Here's how the part is built. I have some questions about the finished solid (model axes, mm). A direction names the side the tool comes from. Coordinates: 2 decimals unless noted, no trailing zeros. Order: outer loops, then holes, each group sorted by start corner. A loop starts at its lowest first (then second) coordinate and runs counter-clockwise, first axis right, second up. Notation, with made-up numbers: (35, 20.25) - (78, 20.25) arc R17 cw to (78, 51.25) - close; hole circle Ø11 at (-38.75, 9). An arc over 180 degrees is marked (long way). Answer in a Markdown table with one row per item. Add a question column.
Item 1: Thinking about a two-plate mould opening in X: for faces 3 (the flat face through (-72.283, -3.131, 117.315)), 4 (the cylindrical face through (-72.839, -3.219, 88.523)), 5 (the flat face through (71.426, -3.131, 119.51)), 6 (the flat face through (-1, -3, 200)), which applies, +X half, -X half, draft (parallel to the pull), parting line (faces both ways), or undercut?
Item 2: I want a section at D-D (y = -3.25). Count the separate pieces of the cut face and the enclosed holes in it, plus the area to 3 significant figures.
Item 3: If I drill on line 1 along X through (y, z) = (-1.75, 90); line 2 along X through (y, z) = (-1.5, 16.5); line 3 along X through (y, z) = (-0.75, -13), over which ranges is the centre line in solid material (lowest first)? Write a range as from..to.
Item 4: On a 3-axis mill with a long thin cutter (end or side, diameter ignored), from which of +Z, -Z, +X, -X, +Y, -Y can I reach the whole of each face in a straight line? I mean faces 1 (the flat face through (-2, 0, 77)), 2 (the flat face through (0, -3, 170)). Say none if no direction works.
Item 5: I want a section at B-B (z = 133). Please give me the cut outline in (x, y), plus the area to 3 significant figures.
Item 6: Will these pins go through, and if not, where does the flat tip stop? pin 1 Ø4 at (x, z) = (-30, 190) entering from +Y; pin 2 Ø6.5 at (x, z) = (70.64, 70.64) entering from -Y; pin 3 Ø3 at (x, y) = (-62, -2) entering from -Z; pin 4 Ø1 at (y, z) = (-4, 37.5) entering from +X.
Item 7: I want a section at C-C (z = -15.5). Please give me the cut outline in (x, y), plus the area to 3 significant figures.
Item 8: I want a section at A-A (x = 0). Please give me the cut outline in (y, z), plus the area to 3 significant figures.
```python
from build123d import *

# Parameters (mm, degrees)
BOSS_EXTRUDE1_DEPTH         = 6.35
M6_CLEARANCE_HOLE1_D        = 6.4
TAP_DRILL_FOR_M6X1_0_TAP1_D = 5
FILLET1_R                   = 5
FILLET2_R                   = 5


with BuildPart() as part:
    # Sketch1 → Boss-Extrude1 (new body)
    with BuildSketch(Plane(origin=(0, 0, 0), x_dir=(1, 0, 0), z_dir=(0, 1, 0))):
        with BuildLine():
            Line((-102.466925197, -40.006614961), (-40, -200))
            Line((-40, -200), (40, -200))
            Line((40, -200), (102.466925197, -40.006614961))
            ThreePointArc((102.466925197, -40.006614961), (0, 110), (-102.466925197, -40.006614961))
        make_face()
        with BuildLine():
            Line((-30, -170), (30, -170))
            Line((30, -170), (62.79649165, -86))
            ThreePointArc((62.79649165, -86), (0, -77.984711576), (-62.79649165, -86))
            Line((-62.79649165, -86), (-30, -170))
        make_face(mode=Mode.SUBTRACT)
        with BuildLine():
            ThreePointArc((-46.479429348, -62.015422658), (0, -57.984711576), (46.479429348, -62.015422658))
            ThreePointArc((46.479429348, -62.015422658), (0, 77.5), (-46.479429348, -62.015422658))
        make_face(mode=Mode.SUBTRACT)
    extrude(amount=-BOSS_EXTRUDE1_DEPTH)

    # M6 Clearance Hole1 (through all)
    with Locations(Plane(origin=(-70, 0, 90), x_dir=(0, 0, 1), z_dir=(0, 1, 0))):
        with Locations((0, 0), (100, 40), (100, 100), (0, 140)):
            Hole(M6_CLEARANCE_HOLE1_D / 2)

    # Tap Drill for M6x1.0 Tap1 (through all)
    with Locations(Plane(origin=(-70.64375, 0, 70.64375), x_dir=(0, 0, 1), z_dir=(0, 1, 0))):
        with Locations((0, 0), (-141.2875, 0), (-141.2875, 141.2875), (0, 141.2875)):
            Hole(TAP_DRILL_FOR_M6X1_0_TAP1_D / 2)

    # Fillet1
    fillet1_edges = [part.edges().sort_by_distance(p)[0] for p in [
        (-46.479429348, -3.175, 62.015422658),
        (46.479429348, -3.175, 62.015422658),
        (-30, -3.175, 170),
        (-62.79649165, -3.175, 86),
        (62.79649165, -3.175, 86),
        (30, -3.175, 170),
    ]]
    fillet(fillet1_edges, radius=FILLET1_R)

    # Fillet2
    fillet2_edges = [part.edges().sort_by_distance(p)[0] for p in [
        (40, -3.175, 200),
        (-40, -3.175, 200),
    ]]
    fillet(fillet2_edges, radius=FILLET2_R)


solid = part.part
```
Values follow:
| question | item | result |
|---|---|---|
| 1 | face 3 | -X half |
| 1 | face 4 | undercut |
| 1 | face 5 | +X half |
| 1 | face 6 | draft |
| 2 | separate pieces | 1 |
| 2 | enclosed holes | 10 |
| 2 | area | 24,100 mm^2 |
| 3 | line 1 | x = -82.95..-73.2, -66.8..-61.04, 61.04..66.8, 73.2..82.95 |
| 3 | line 2 | x = -108.76..-75.72, 75.72..108.76 |
| 3 | line 3 | x = -109.23..-76.4, 76.4..109.23 |
| 4 | face 1 | +Z, -Z, +X, -X, +Y |
| 4 | face 2 | +Y, -Y |
| 5 | outline | (-66.16, -6.35) - (-44.45, -6.35) - (-44.45, 0) - (-66.16, 0) - close; (44.45, -6.35) - (66.16, -6.35) - (66.16, 0) - (44.45, 0) - close |
| 5 | area | 276 mm^2 |
| 6 | pin 1 | passes through |
| 6 | pin 2 | stops at y = -6.35 |
| 6 | pin 3 | stops at z = -91.87 |
| 6 | pin 4 | stops at x = 103.59 |
| 7 | outline | (-108.9, -6.35) - (-75.93, -6.35) - (-75.93, 0) - (-108.9, 0) - close; (75.93, -6.35) - (108.9, -6.35) - (108.9, 0) - (75.93, 0) - close |
| 7 | area | 419 mm^2 |
| 8 | outline | (-6.35, -110) - (0, -110) - (0, -77.5) - (-6.35, -77.5) - close; (-6.35, 57.98) - (0, 57.98) - (0, 77.98) - (-6.35, 77.98) - close; (-6.35, 170) - (0, 170) - (0, 200) - (-6.35, 200) - close |
| 8 | area | 524 mm^2 |
